Here's how the part is built. I have some questions about the finished solid (model axes, mm). A direction names the side the tool comes from. Coordinates: 2 decimals unless noted, no trailing zeros. Write each loop counter-clockwise with the first axis right and the second up, starting at its lowest first coordinate (ties: lowest second). Pieces come first, ordered by that corner, then holes.
Item 1: If we section it at A-A (x = -63): Please give me the cut outline in (y, z) (3 decimals).
Item 2: If we section it at B-B (y = 5.75): Please give me the cut outline in (x, z).
Item 3: I'm going to push flat-ended pins straight in: pin 1 Ø1.5 at (y, z) = (6, 3) entering from +X; pin 2 Ø3 at (x, y) = (-153.5, -4.5) entering from +Z; pin 3 Ø3 at (x, z) = (-161.5, -3) entering from -Y. Where does each tip first touch, or does it pass through?
Item 4: For faces 1 (the face through (-6.26, 1.93, -2.52)), 2 (the face through (-137.92, 9.3, -2.06)), which set-ups out of +Z, -Z, +X, -X, +Y, -Y let a thin tool reach every point of the face, with its end or its side?
Item 5: If I drill on line 1 (Y direction, x = -262.75, z = 0) (3 decimals); line 2 (Z direction, x = -13, y = -1); line 3 (X direction, y = -5, z = -1.75), over which ranges is the centre line in solid material (lowest first)?
from build123d import *

# Parameters (mm, degrees)
SKETCH2_R          = 0.79375
CUT_EXTRUDE1_DEPTH = 12.7


with BuildPart() as part:
    # Sketch1 → Revolve1 (revolve)
    with BuildSketch(Plane.XY, mode=Mode.PRIVATE) as revolve1_sk:
        Polygon((-266.7, 0), (-266.7, 9.525), (-12.7, 9.525), (-12.7, 3.175), (0, 3.175), (0, 0), align=None)
    revolve(revolve1_sk.sketch.rotate(Axis((-54.16626506, 0, 0), (1, 0, 0)), 90), axis=Axis((-54.16626506, 0, 0), (1, 0, 0)))

    # Sketch2 → Cut-Extrude1 (cut)
    with BuildSketch(Plane.ZY.offset(266.7)):
        Circle(SKETCH2_R)
    extrude(amount=-CUT_EXTRUDE1_DEPTH, mode=Mode.SUBTRACT)


solid = part.part
Answer list:
1. outline: circle Ø19.05 at (0, 0)
2. outline: (-266.7, -7.59) - (-12.7, -7.59) - (-12.7, 7.59) - (-266.7, 7.59) - close
3. pin 1: stops at x = -12.7
3. pin 2: stops at z = 9.04
3. pin 3: stops at y = -9.41
4. face 1: +X
4. face 2: +X, -X
5. line 1: y = -9.525 to -0.794, 0.794 to 9.525
5. line 2: z = -9.47 to 9.47
5. line 3: x = -266.7 to -12.7
